Could you check a few things on this drawing? It's one solid part, dimensions in mm from its lowest x, y, z. A direction names the side the tool comes from. Give positions to 0.01 mm unless a question says otherwise; leave off trailing zeros. Order: outer loops, then holes, each group sorted by start corner. A loop starts at its lowest first (then second) coordinate and runs counter-clockwise, first axis right, second up. Notation, with made-up numbers: (58.25, 38.25) -> (107.25, 38.25) arc R22 ccw to (107.25, 48.25) -> close; hole circle Ø1 at (74.25, -29). An arc over 180 degrees is marked (long way). Answer as CSV lines item,"result".
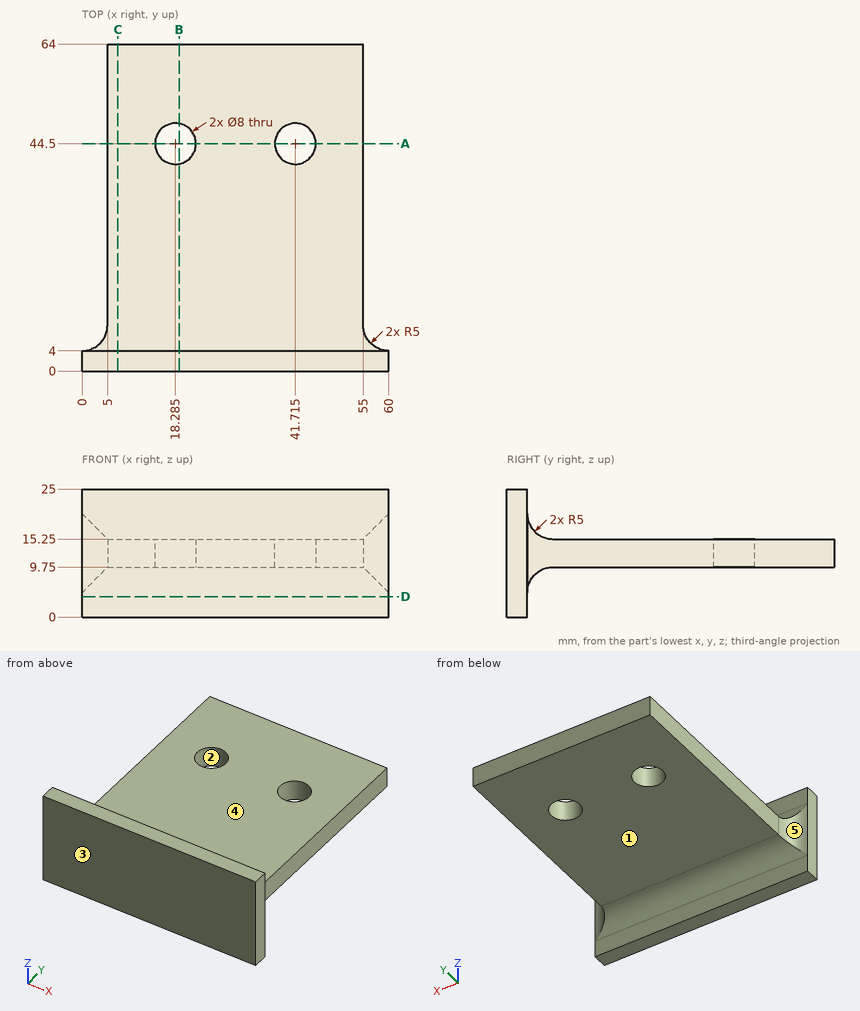
Item 1: Imagine slicing it at D-D, the plane z = 4. Please give me the cut outline in (x, y).
Numbers:
outline,"(0, 0) -> (60, 0) -> (60, 4) -> (0, 4) -> close"
Item 2: Imagine slicing it at A-A, the plane y = 44.5. Please give me the cut outline in (x, z) (3 decimals), then the cut area to 3 significant figures.
Numbers:
outline,"(5, 9.75) -> (14.285, 9.75) -> (14.285, 15.25) -> (5, 15.25) -> close; (22.285, 9.75) -> (37.715, 9.75) -> (37.715, 15.25) -> (22.285, 15.25) -> close; (45.715, 9.75) -> (55, 9.75) -> (55, 15.25) -> (45.715, 15.25) -> close"
area,"187 mm²"
Item 3: We'd pull the mould along Y, two halves only. Please class the marked faces 1, 2 and 3: released by +Y, released by -Y, zero draft, split by the parting line, or undercut.
Numbers:
face 1,"zero draft"
face 2,"undercut"
face 3,"released by -Y"
Item 4: For the marked faces 4 and 5, which set-ups out of +Z, -Z, +X, -X, +Y, -Y let a thin tool reach every point of the face, with its end or its side?
Numbers:
face 4,"+Z, +X, -X, +Y"
face 5,"+Z, -Z, -X, +Y"
Item 5: Imagine slicing it at B-B, the plane x = 19. Please give me the cut outline in (y, z).
Numbers:
outline,"(0, 0) -> (4, 0) -> (4, 4.75) arc R5 cw to (9, 9.75) -> (40.56, 9.75) -> (40.56, 15.25) -> (9, 15.25) arc R5 cw to (4, 20.25) -> (4, 25) -> (0, 25) -> close; (48.44, 9.75) -> (64, 9.75) -> (64, 15.25) -> (48.44, 15.25) -> close"
Item 6: Imagine slicing it at C-C, the plane x = 7. Please give me the cut outline in (y, z), then the cut area to 3 significant figures.
Numbers:
outline,"(0, 0) -> (4, 0) -> (4, 4.75) arc R5 cw to (9, 9.75) -> (64, 9.75) -> (64, 15.25) -> (9, 15.25) arc R5 cw to (4, 20.25) -> (4, 25) -> (0, 25) -> close"
area,"441 mm²"
Item 7: For pin 1 (4 mm diameter, centred on x = 50, y = 44, fed in from +Z); pin 2 (5 mm diameter, centred on x = 30.5, y = 18, fed in from -Z); pin 3 (1.6 mm diameter, centred on y = 26, z = 13, fed in from +X), each with a flat end and sliding along its axis, tell me the tip position at first contact or that it passes through.
Numbers:
pin 1,"stops at z = 15.25"
pin 2,"stops at z = 9.75"
pin 3,"stops at x = 55"
Item 8: Please list where these lines run through material, in increasing order: line 1 along X through (y, z) = (45.5, 13.75); line 2 along Z through (x, y) = (48, 43); line 3 along Y through (x, z) = (7.5, 20.25).
Numbers:
line 1,"x = 5 to 14.41, 22.16 to 37.84, 45.59 to 55"
line 2,"z = 9.75 to 15.25"
line 3,"y = 0 to 4"
